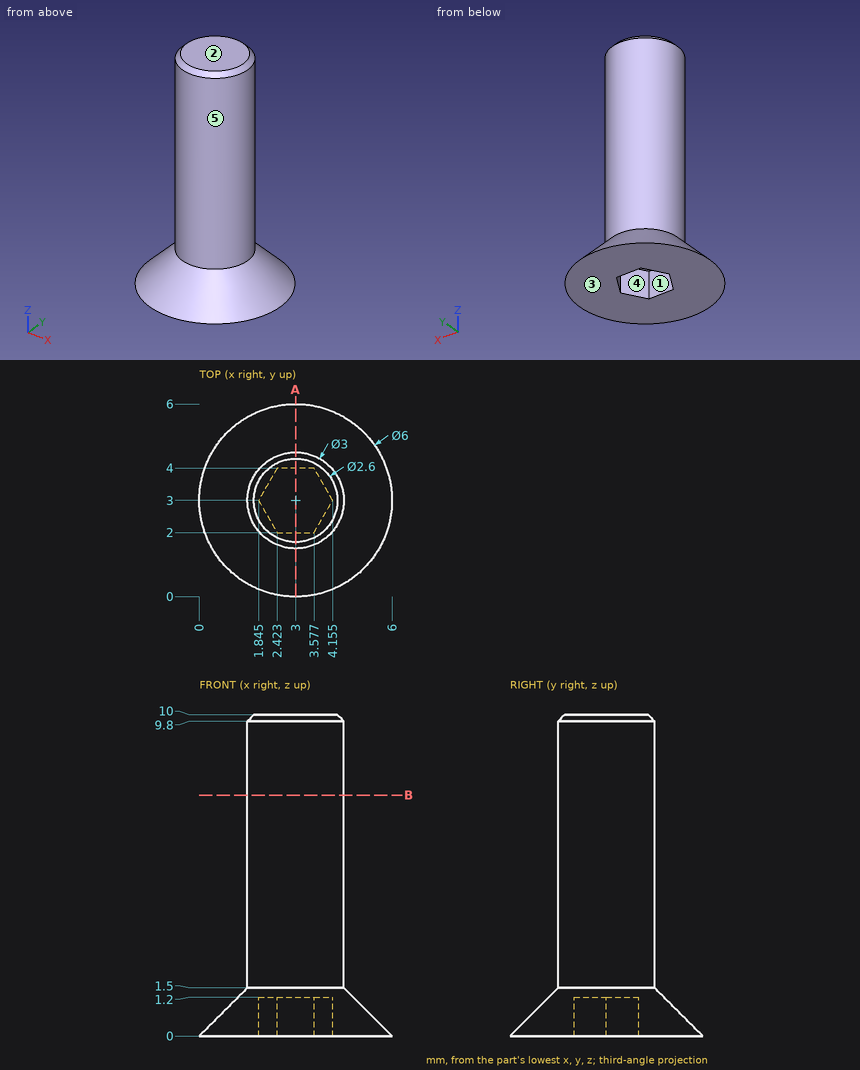
Design review of the part shown in the three views and the two pictorial views. Dimensions are in mm from the part's minimum x, y and z. A direction names the side the tool comes from. Give positions to 0.01 mm unless a question says otherwise; leave off trailing zeros. Loops run counter-clockwise (first coordinate to the right, second up) from the corner with the lowest first, then second, coordinate; pieces in that order, holes last. Notation, with made-up numbers: M 10,-9.5 L 55,-9.5 A24 ccw 55,5.5 Z; hole C -22.5,39.25 d8. An arc over 180 degrees is marked long. Write item = value, one per line.
Q1. Insertion check: pin 1 (0.9 mm diameter, centred on x = 3, z = 0.5, fed in from +Y). The pin has a flat end and moves straight along its axis. Give the tip position at first contact, or say it passes through.
Output values:
pin_1 = 5.95
Q2. We need section A-A (x = 3). Give the boundary of the cut face in (y, z), plus the area to 3 significant figures.
Output values:
outline = M 0,0 L 2,0 L 2,1.2 L 4,1.2 L 4,0 L 6,0 L 4.5,1.5 L 4.5,9.8 L 4.3,10 L 1.7,10 L 1.5,9.8 L 1.5,1.5 Z
area = 29.8 mm^2
Q3. We need section B-B (z = 7.5). Give the boundary of the cut face in (x, y).
Output values:
outline = C 3,3 d3
Q4. Draft analysis for pull direction X (two halves, no side actions). For the marked faces 3, 4 and 5, state which applies: +X half, -X half, draft (parallel to the pull), parting line (faces both ways), or undercut.
Output values:
face_3 = draft
face_4 = undercut
face_5 = parting line
Q5. For the marked faces 1 and 2, list the 3-axis set-ups (+Z, -Z, +X, -X, +Y, -Y) from which the entire face can be reached by the end or side of a thin tool; tool diameter is ignored.
Output values:
face_1 = -Z
face_2 = +Z, +X, -X, +Y, -Y
Q6. To check wall thickness, follow line 1 (Z direction, x = 2.9, y = 2.25); line 2 (Y direction, x = 3.05, z = 7.5); line 3 (Z direction, x = 3.75, y = 4.8). State the ranges of each line that lie inside material, in increasing order. Write a range as [from, to].
Output values:
line_1 = [1.2, 10]
line_2 = [1.5, 4.5]
line_3 = [0, 1.05]
